Build history of the part. All positions in model axes, mm. A direction names the side the tool comes from. Give positions to 0.01 mm unless a question says otherwise; leave off trailing zeros. Order: outer loops, then holes, each group sorted by start corner. A loop starts at its lowest first (then second) coordinate and runs counter-clockwise, first axis right, second up. Notation, with made-up numbers: (-32, -13.75) -> (24, -13.75) arc R12 cw to (24, -5.75) -> close; hole circle Ø8 at (4, 41). An arc over 180 degrees is marked (long way). Use a Markdown table: item, result. Add a question column.
```python
from build123d import *

# Parameters (mm, degrees)
BOSS_EXTRU_1_DEPTH      = 22
ESQUISSE2_R             = 1.7
ENL_V_MAT_EXTRU_1_DEPTH = 23
ESQUISSE3_R             = 9
ESQUISSE3_R_2           = 1.3
BOSS_EXTRU_2_DEPTH      = 14
ESQUISSE4_W             = 0.84262724
ESQUISSE4_H             = 4.751474998
ENL_V_MAT_EXTRU_2_DEPTH = 12
ESQUISSE5_R             = 1.3
ENL_V_MAT_EXTRU_3_DEPTH = 27
ESQUISSE6_R             = 2.1
ENL_V_MAT_EXTRU_4_DEPTH = 14


with BuildPart() as part:
    # Esquisse1 → Boss.-Extru.1 (new body)
    with BuildSketch(Plane.XY):
        Polygon((6, 3.464101615), (0, 6.92820323), (-6, 3.464101615), (-6, -3.464101615), (0, -6.92820323), (6, -3.464101615), align=None)
    extrude(amount=BOSS_EXTRU_1_DEPTH)

    # Esquisse2 → Enlèv. mat.-Extru.1 (cut)
    with BuildSketch(Plane.XY.offset(22)):
        Circle(ESQUISSE2_R)
    extrude(amount=-ENL_V_MAT_EXTRU_1_DEPTH, mode=Mode.SUBTRACT)

    # Esquisse3 → Boss.-Extru.2 (add)
    with BuildSketch(Plane.XY.offset(22)):
        Circle(ESQUISSE3_R)
        Circle(ESQUISSE3_R_2, mode=Mode.SUBTRACT)
    extrude(amount=-BOSS_EXTRU_2_DEPTH)

    # Esquisse4 → Enlèv. mat.-Extru.2 (cut)
    with BuildSketch(Plane.XY.offset(22)):
        with Locations((9, 0)):
            Rectangle(ESQUISSE4_W, ESQUISSE4_H)
    extrude(amount=-ENL_V_MAT_EXTRU_2_DEPTH, mode=Mode.SUBTRACT)

    # Esquisse5 → Enlèv. mat.-Extru.3 (cut)
    with BuildSketch(Plane(origin=(8.57868638, 0, 0), x_dir=(0, 0, -1), z_dir=(1, 0, 0))):
        with Locations((-15, 0)):
            Circle(ESQUISSE5_R)
    extrude(amount=-ENL_V_MAT_EXTRU_3_DEPTH, mode=Mode.SUBTRACT)

    # Esquisse6 → Enlèv. mat.-Extru.4 (cut)
    with BuildSketch(Plane.XY.offset(22)):
        Circle(ESQUISSE6_R)
    extrude(amount=-ENL_V_MAT_EXTRU_4_DEPTH, mode=Mode.SUBTRACT)


solid = part.part
```
(1) Mould opens along Y. For faces 4 (the face through (-2.25, 0.13, 22)), 5 (the face through (-5.27, 0.06, 16.3)), 6 (the face through (-2.96, 5.22, 3.94)) say: released by +Y, released by -Y, zero draft, split by the parting line, or undercut.
(2) Pin check, flat tips, straight feed: pin 1 Ø2 at (x, z) = (4, 4.5) entering from +Y; pin 2 Ø3.5 at (y, z) = (1.5, 3) entering from +X; pin 3 Ø1.4 at (y, z) = (1, 18) entering from +X. Stop position of each tip, or through.
(3) Band-saw the part on C-C on x = -3.75. Give the cut face in (y, z), plus the area to 3 significant figures.
(4) Band-saw the part on B-B on z = 5. Give the cut face in (x, y).
(5) Tool access for faces 1 (the face through (-0.273, 2.082, 15.098)), 2 (the face through (-3.042, -5.172, 3.944)), 3 (the face through (3.042, 5.172, 3.944)): list every direction of +Z, -Z, +X, -X, +Y, -Y with a clear straight run to the whole face (end or side of a thin tool).
(6) Band-saw the part on D-D on x = -0.75. Give the cut face in (y, z).
(7) Band-saw the part on A-A on y = 0. Give the cut face in (x, z), plus the area to 3 significant figures.
(8) Wall check: probe 1 along Y at (x, z) = (0, 13.5); probe 2 along Z at (x, y) = (3.25, 0); probe 3 along Y at (x, z) = (-0.5, 18.75). Give the ranges that are in metal, low to high.
Response:
| question | item | result |
|---|---|---|
| 1 | face 4 | zero draft |
| 1 | face 5 | undercut |
| 1 | face 6 | released by +Y |
| 2 | pin 1 | stops at y = 5.2 |
| 2 | pin 2 | stops at x = 6 |
| 2 | pin 3 | stops at x = 8.58 |
| 3 | outline | (-8.18, 8) -> (-4.76, 8) -> (-4.76, 0) -> (4.76, 0) -> (4.76, 8) -> (8.18, 8) -> (8.18, 22) -> (-8.18, 22) -> close; hole circle Ø2.6 at (0, 15) |
| 3 | area | 300 mm² |
| 4 | outline | (-6, -3.46) -> (0, -6.93) -> (6, -3.46) -> (6, 3.46) -> (0, 6.93) -> (-6, 3.46) -> close; hole circle Ø3.4 at (0, 0) |
| 5 | face 1 | +Z |
| 5 | face 2 | -Z, -X, -Y |
| 5 | face 3 | -Z, +X, +Y |
| 6 | outline | (-8.97, 8) -> (-6.5, 8) -> (-6.5, 0) -> (-1.53, 0) -> (-1.53, 8) -> (-1.96, 8) -> (-1.96, 22) -> (-8.97, 22) -> close; (1.53, 0) -> (6.5, 0) -> (6.5, 8) -> (8.97, 8) -> (8.97, 22) -> (1.96, 22) -> (1.96, 8) -> (1.53, 8) -> close |
| 7 | outline | (-9, 8) -> (-6, 8) -> (-6, 0) -> (-1.7, 0) -> (-1.7, 8) -> (-2.1, 8) -> (-2.1, 13.7) -> (-9, 13.7) -> close; (-9, 16.3) -> (-2.1, 16.3) -> (-2.1, 22) -> (-9, 22) -> close; (1.7, 0) -> (6, 0) -> (6, 8) -> (9, 8) -> (9, 10) -> (8.58, 10) -> (8.58, 13.7) -> (2.1, 13.7) -> (2.1, 8) -> (1.7, 8) -> close; (2.1, 16.3) -> (8.58, 16.3) -> (8.58, 22) -> (2.1, 22) -> close |
| 7 | area | 222 mm² |
| 8 | probe 1 | y = -9 to -2.1, 2.1 to 9 |
| 8 | probe 2 | z = 0 to 13.7, 16.3 to 22 |
| 8 | probe 3 | y = -8.99 to -2.04, 2.04 to 8.99 |
